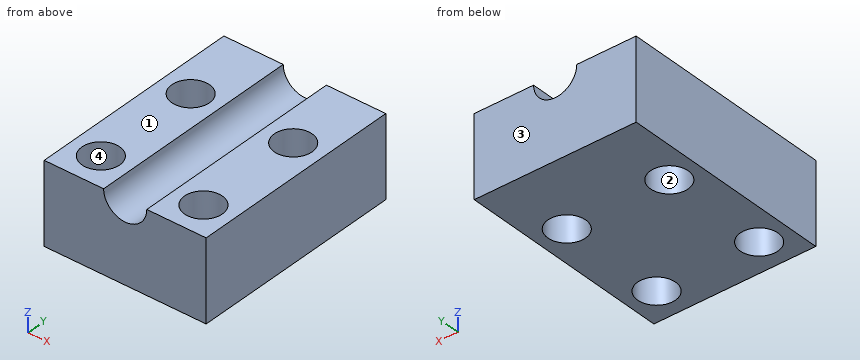
```python
from build123d import *

# Parameters (mm, degrees)
F0_W     = 30
F0_H     = 40
F1_DEPTH = 15
F3_DEPTH = 40
F4_R     = 3.5
F5_DEPTH = 15


with BuildPart() as f1:
    # F0 (on Top) → F1 (new body)
    with BuildSketch(Plane.XY):
        with Locations((0, -20)):
            Rectangle(F0_W, F0_H)
    extrude(amount=F1_DEPTH)

    # F2 (on face) → F3 (cut, through all)
    with BuildSketch(Plane.XZ.offset(40)):
        with BuildLine():
            ThreePointArc((-4, 15), (0, 11), (4, 15))
            Line((4, 15), (-4, 15))
        make_face()
    extrude(amount=-F3_DEPTH, mode=Mode.SUBTRACT)

    # F4 (on face) → F5 (cut, through all)
    with BuildSketch(Plane.XY.offset(15)):
        with Locations((-9.5, -34)):
            Circle(F4_R)
        with Locations((-9.5, -14)):
            Circle(F4_R)
        with Locations((9.5, -14)):
            Circle(F4_R)
        with Locations((9.5, -34)):
            Circle(F4_R)
    extrude(amount=-F5_DEPTH, mode=Mode.SUBTRACT)


solid = f1.part
```
The listing builds one solid part. Answer for the finished solid, in the listing's coordinates (mm). Face numbers are marked on the shaded views. Coordinates: 2 decimals unless noted, no trailing zeros. Write each loop counter-clockwise with the first axis right and the second up, starting at its lowest first coordinate (ties: lowest second). Pieces come first, ordered by that corner, then holes. Notation, with made-up numbers: (25.5, 32.25) -> (51.5, 32.25) arc R26 cw to (51.5, 56.25) -> close; hole circle Ø6 at (84, 81.5). An arc over 180 degrees is marked (long way). Write each question's results on one line, items separated by ' | '. Start each with the question number.
1) A cutting plane is placed at C-C (y = -8). Determine the outline of the cut face in (x, z), then the cut area to 3 significant figures.
2) A cutting plane is placed at D-D (x = 10.5). Determine the outline of the cut face in (y, z).
3) A flat-ended cylindrical pin translates along its axis: pin 1 Ø1.5 at (x, y) = (-1, -12.5) entering from +Z. Find the tip coordinate at first contact, or state that the pin passes through.
4) For a pull along Y with two mould halves and no side action, classify the marked faces 1, 2, 3 and 4 as +Y half, -Y half, draft (parallel to the pull), parting line (faces both ways), or undercut.
5) A cutting plane is placed at A-A (y = -34). Determine the outline of the cut face in (x, z).
6) Straight lines are drawn through the part: probe 1 along Y at (x, z) = (9.5, 11.5); probe 2 along X at (y, z) = (-35.5, 10.5); probe 3 along Y at (x, z) = (10.25, 5.5). For each, find the intervals that lie inside material, in ascending order.
7) A cutting plane is placed at B-B (z = 1.5). Determine the outline of the cut face in (x, y), then the cut area to 3 significant figures.
Values follow:
1) outline: (-15, 0) -> (15, 0) -> (15, 15) -> (4, 15) arc R4 cw to (-4, 15) -> (-15, 15) -> close | area: 425 mm²
2) outline: (-40, 0) -> (-37.35, 0) -> (-37.35, 15) -> (-40, 15) -> close; (-30.65, 0) -> (-17.35, 0) -> (-17.35, 15) -> (-30.65, 15) -> close; (-10.65, 0) -> (0, 0) -> (0, 15) -> (-10.65, 15) -> close
3) pin 1: z = 11.4
4) face 1: draft | face 2: undercut | face 3: +Y half | face 4: undercut
5) outline: (-15, 0) -> (-13, 0) -> (-13, 15) -> (-15, 15) -> close; (-6, 0) -> (6, 0) -> (6, 15) -> (4, 15) arc R4 cw to (-4, 15) -> (-6, 15) -> close; (13, 0) -> (15, 0) -> (15, 15) -> (13, 15) -> close
6) probe 1: -40 to -37.5, -30.5 to -17.5, -10.5 to 0 | probe 2: -15 to -12.66, -6.34 to 6.34, 12.66 to 15 | probe 3: -40 to -37.42, -30.58 to -17.42, -10.58 to 0
7) outline: (-15, -40) -> (15, -40) -> (15, 0) -> (-15, 0) -> close; hole circle Ø7 at (-9.5, -34); hole circle Ø7 at (-9.5, -14); hole circle Ø7 at (9.5, -34); hole circle Ø7 at (9.5, -14) | area: 1,050 mm²
